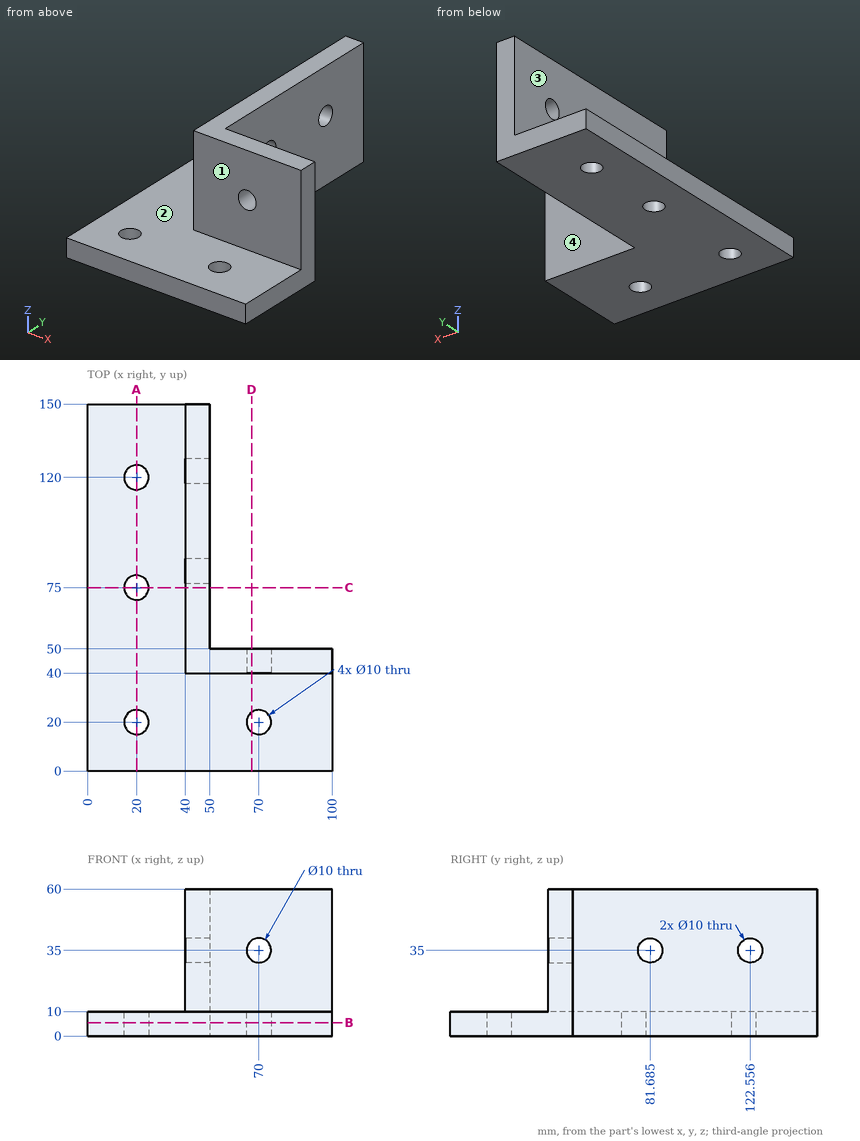
Study the drawing (mm; zero at the part's minimum x, y, z) and answer. A direction names the side the tool comes from. Round coordinates to 2 decimals unless told otherwise and drop trailing zeros. Write each loop counter-clockwise with the first axis right and the second up, starting at its lowest first coordinate (ties: lowest second). Pieces come first, ordered by that corner, then holes.
Q1. Flat-ended cylindrical pins translate along their axes: P1, Ø9, axis at x = 70, y = 20, coming from the +Z side; P2, Ø1, axis at x = 53.5, y = 21.5, coming from the +Z side; P3, Ø10, axis at y = 112.5, z = 50.5, coming from the +X side; P4, Ø25, axis at x = 80.5, z = 23.5, coming from the -Y side. Find the tip coordinate at first contact, or state that the pin passes through.
Values:
P1: passes through
P2: stops at z = 10
P3: stops at x = 50
P4: stops at y = 40
Q2. Find section A-A on x = 20. Determine the outline of the cut face in (y, z), and give its area (3 significant figures).
Values:
outline: (0, 0) - (15, 0) - (15, 10) - (0, 10) - close; (25, 0) - (70, 0) - (70, 10) - (25, 10) - close; (80, 0) - (115, 0) - (115, 10) - (80, 10) - close; (125, 0) - (150, 0) - (150, 10) - (125, 10) - close
area: 1,200 mm2
Q3. Find section C-C on y = 75. Determine the outline of the cut face in (x, z).
Values:
outline: (0, 0) - (15, 0) - (15, 10) - (0, 10) - close; (25, 0) - (50, 0) - (50, 60) - (40, 60) - (40, 10) - (25, 10) - close
Q4. Find section D-D on x = 67. Determine the outline of the cut face in (y, z), and give its area (3 significant figures).
Values:
outline: (0, 0) - (16, 0) - (16, 10) - (0, 10) - close; (24, 0) - (50, 0) - (50, 31) - (40, 31) - (40, 10) - (24, 10) - close; (40, 39) - (50, 39) - (50, 60) - (40, 60) - close
area: 840 mm2
Q5. A tool of negligible diameter and unlimited length cuts with its end or side. For the marked faces 1, 2, 3 and 4, from which of +Z, -Z, +X, -X, +Y, -Y can it reach the whole face along a straight path? Write none if from no direction.
Values:
face 1: +Z, +X, -X, -Y
face 2: +Z, -X, -Y
face 3: +Z, -X, +Y, -Y
face 4: +Z, -Z, +X, +Y
Q6. Straight lines are drawn through the part: line 1 (Y direction, x = 20, z = 7); line 2 (Y direction, x = 70, z = 7.25); line 3 (X direction, y = 44, z = 35). For each, find the intervals that lie inside material, in ascending order.
Values:
line 1: y = 0 to 15, 25 to 70, 80 to 115, 125 to 150
line 2: y = 0 to 15, 25 to 50
line 3: x = 40 to 65, 75 to 100
Q7. Find section B-B on z = 5.5. Determine the outline of the cut face in (x, y).
Values:
outline: (0, 0) - (100, 0) - (100, 50) - (50, 50) - (50, 150) - (0, 150) - close; hole circle Ø10 at (20, 20); hole circle Ø10 at (20, 75); hole circle Ø10 at (20, 120); hole circle Ø10 at (70, 20)
